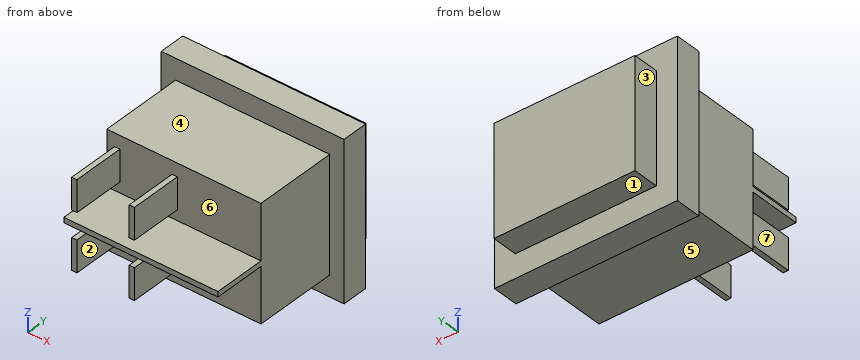
from build123d import *

# Parameters (mm, degrees)
SKETCH_1_W      = 29.5
SKETCH_1_H      = 22
EXTRUDE_1_DEPTH = 16
SKETCH_2_W      = 35
SKETCH_2_H      = 30
EXTRUDE_2_DEPTH = 5
SKETCH_3_W      = 27
SKETCH_3_H      = 21
EXTRUDE_3_DEPTH = 5
SKETCH_4_W      = 29.5
SKETCH_4_H      = 1
SKETCH_4_W_2    = 1
SKETCH_4_H_2    = 6
EXTRUDE_4_DEPTH = 10


with BuildPart() as part:
    # Эскиз1 → Бобышка-Вытянуть1 (new body)
    with BuildSketch(Plane(origin=(0, 0, 0), x_dir=(1, 0, 0), z_dir=(0, 1, 0))):
        Rectangle(SKETCH_1_W, SKETCH_1_H)
    extrude(amount=-EXTRUDE_1_DEPTH)

    # Эскиз2 → Бобышка-Вытянуть2 (add)
    with BuildSketch(Plane(origin=(0, 0, 0), x_dir=(1, 0, 0), z_dir=(0, 1, 0))):
        Rectangle(SKETCH_2_W, SKETCH_2_H)
    extrude(amount=EXTRUDE_2_DEPTH)

    # Эскиз3 → Бобышка-Вытянуть3 (add)
    with BuildSketch(Plane(origin=(0, 5, 0), x_dir=(1, 0, 0), z_dir=(0, 1, 0))):
        Rectangle(SKETCH_3_W, SKETCH_3_H)
    extrude(amount=EXTRUDE_3_DEPTH)

    # Эскиз4 → Бобышка-Вытянуть4 (add)
    with BuildSketch(Plane.XZ.offset(16)):
        Rectangle(SKETCH_4_W, SKETCH_4_H)
        with Locations((-12.75, 5.5)):
            Rectangle(SKETCH_4_W_2, SKETCH_4_H_2)
        with Locations((-1.75, 5.5)):
            Rectangle(SKETCH_4_W_2, SKETCH_4_H_2)
        with Locations((-12.75, -5.5)):
            Rectangle(SKETCH_4_W_2, SKETCH_4_H_2)
        with Locations((-1.75, -5.5)):
            Rectangle(SKETCH_4_W_2, SKETCH_4_H_2)
    extrude(amount=EXTRUDE_4_DEPTH)


solid = part.part
Design review of the part built by this model. Coordinates are the model's own, in mm. Face numbers are marked on the shaded views. A direction names the side the tool comes from. Round coordinates to 2 decimals unless told otherwise and drop trailing zeros. Loops run counter-clockwise (first coordinate to the right, second up) from the corner with the lowest first, then second, coordinate; pieces in that order, holes last. Notation, with made-up numbers: (83, 32) - (140, 32) arc R31 cw to (140, 70) - close; hole circle Ø7 at (80, 69.25). An arc over 180 degrees is marked (long way). One line per item, written item: value. Start each with the question number.
1) For the marked faces 1, 2, 3 and 4, list the 3-axis set-ups (+Z, -Z, +X, -X, +Y, -Y) from which the entire face can be reached by the end or side of a thin tool; tool diameter is ignored.
2) Consider section B-B on z = 1.5. Give the boundary of the cut face in (x, y), then the cut area to 3 significant figures.
3) Consider section A-A on y = -19.5. Give the boundary of the cut face in (x, z), then the cut area to 3 significant figures.
4) Consider section D-D on y = -8.5. Give the boundary of the cut face in (x, z).
5) To check wall thickness, follow L1, parallel to X at y = -23.5, z = 4.5; L2, parallel to X at y = -10, z = 5.75; L3, parallel to Y at x = 10, z = 2.75. State the ranges of each line that lie inside material, in increasing order. Write a range as from..to.
6) Insertion check: pin 1 Ø5.5 at (x, y) = (-6, 8) entering from +Z; pin 2 Ø8 at (x, y) = (-4, -5.5) entering from -Z; pin 3 Ø0.5 at (x, y) = (-12.5, -22) entering from +Z. Each pin has a flat end and moves straight along its axis. Give the tip position at first contact, or say it passes through.
7) Draft analysis for pull direction X (two halves, no side actions). For the marked faces 5, 6 and 7, state which applies: +X half, -X half, draft (parallel to the pull), parting line (faces both ways), or undercut.
8) Consider section C-C on x = -0.5. Give the boundary of the cut face in (y, z), then the cut area to 3 significant figures.
Reported:
1. face 1: -Z, +X, -X, +Y
1. face 2: -Z, -Y
1. face 3: +Z, -Z, -X, +Y
1. face 4: +Z, +X, -X, -Y
2. outline: (-17.5, 0) - (-14.75, 0) - (-14.75, -16) - (14.75, -16) - (14.75, 0) - (17.5, 0) - (17.5, 5) - (13.5, 5) - (13.5, 10) - (-13.5, 10) - (-13.5, 5) - (-17.5, 5) - close
2. area: 782 mm^2
3. outline: (-14.75, -0.5) - (14.75, -0.5) - (14.75, 0.5) - (-14.75, 0.5) - close; (-13.25, -8.5) - (-12.25, -8.5) - (-12.25, -2.5) - (-13.25, -2.5) - close; (-13.25, 2.5) - (-12.25, 2.5) - (-12.25, 8.5) - (-13.25, 8.5) - close; (-2.25, -8.5) - (-1.25, -8.5) - (-1.25, -2.5) - (-2.25, -2.5) - close; (-2.25, 2.5) - (-1.25, 2.5) - (-1.25, 8.5) - (-2.25, 8.5) - close
3. area: 53.5 mm^2
4. outline: (-14.75, -11) - (14.75, -11) - (14.75, 11) - (-14.75, 11) - close
5. L1: x = -13.25..-12.25, -2.25..-1.25
5. L2: x = -14.75..14.75
5. L3: y = -16..10
6. pin 1: stops at z = 10.5
6. pin 2: stops at z = -11
6. pin 3: stops at z = 8.5
7. face 5: draft
7. face 6: undercut
7. face 7: -X half
8. outline: (-26, -0.5) - (-16, -0.5) - (-16, -11) - (0, -11) - (0, -15) - (5, -15) - (5, -10.5) - (10, -10.5) - (10, 10.5) - (5, 10.5) - (5, 15) - (0, 15) - (0, 11) - (-16, 11) - (-16, 0.5) - (-26, 0.5) - close
8. area: 617 mm^2
